```python
from build123d import *

# Parameters (mm, degrees)
SKETCH_W             = 18
SKETCH_H             = 25.7
PAD001_DEPTH         = 1
SKETCH002_R          = 1.1
PAD002_DEPTH         = 4.25
SKETCH004_W          = 20
SKETCH004_H          = 27.7
PAD004_DEPTH         = 8.5
SKETCH005_W          = 16
SKETCH005_H          = 0.5
POCKET_DEPTH         = 13.851
POCKET_DEPTH_BACK    = 13.851
SKETCH006_W          = 23.7
SKETCH006_H          = 0.5
POCKET001_DEPTH      = 10.001
POCKET001_DEPTH_BACK = 10.001
SKETCH007_W          = 18.8
SKETCH007_H          = 26.5
POCKET002_DEPTH      = 1


with BuildPart() as body004:
    # Sketch → Pad001 (new body)
    with BuildSketch(Plane.XY):
        Rectangle(SKETCH_W, SKETCH_H)
    extrude(amount=PAD001_DEPTH)

    # Sketch002 → Pad002 (join)
    with BuildSketch(Plane.XY):
        with Locations((5.556277, -9.06)):
            Circle(SKETCH002_R)
        Polygon((1.664554, 10.16), (1.400063, 8.66), (-2.320768, 8.66), (-2.950092, 9.41), (-2.056277, 10.16), align=None)
        Polygon((1.91841, 10.16), (1.65392, 8.66), (5.343461, 8.66), (6.237276, 9.41), (5.607952, 10.16), align=None)
        Polygon((-3.141603, 9.249303), (-2.512279, 8.499303), (-3.840514, 0.966506), (-4.734329, 0.216506), (-5.317726, 1.226979), (-4.035419, 8.499303), align=None)
        Polygon((6.397973, 9.218489), (5.504158, 8.468489), (4.217444, 1.171169), (4.80084, 0.160697), (5.694655, 0.910697), (7.027298, 8.468489), align=None)
        Polygon((-3.715514, 0.75), (-4.609329, 0), (-4.176316, -0.75), (-0.259174, -0.75), (0.005317, 0.75), align=None)
        Polygon((0.259174, 0.75), (-0.005317, -0.75), (3.715514, -0.75), (4.609329, 0), (4.176316, 0.75), align=None)
        Polygon((4.734329, -0.216506), (3.840514, -0.966506), (2.512279, -8.499303), (3.141603, -9.249303), (4.035419, -8.499303), (5.317726, -1.226979), align=None)
        Polygon((-4.217444, -1.171169), (-4.80084, -0.160697), (-5.694655, -0.910697), (-7.027298, -8.468489), (-6.397973, -9.218489), (-5.504158, -8.468489), align=None)
        Polygon((-5.343461, -8.66), (-6.237276, -9.41), (-5.607952, -10.16), (-1.91841, -10.16), (-1.65392, -8.66), align=None)
        Polygon((-1.400063, -8.66), (-1.664554, -10.16), (2.056277, -10.16), (2.950092, -9.41), (2.320768, -8.66), align=None)
        Polygon((-0.946713, -1.05), (0.576427, -1.05), (-0.712524, -8.36), (-2.235664, -8.36), align=None)
        Polygon((-0.576427, 1.05), (0.946713, 1.05), (2.235664, 8.36), (0.712524, 8.36), align=None)
        Polygon((-2.223397, 8.41), (-2.719177, 5.598295), (-0.889871, 1), (-0.394092, 3.811705), align=None)
        Polygon((1.791361, 4.112606), (1.242525, 1), (4.640381, 5.297394), (5.189217, 8.41), align=None)
        Polygon((0.889871, -1), (0.394092, -3.811705), (2.223397, -8.41), (2.719177, -5.598295), align=None)
        Polygon((-1.242525, -1), (-1.791361, -4.112606), (-5.189217, -8.41), (-4.640381, -5.297394), align=None)
    extrude(amount=PAD002_DEPTH)


with BuildPart() as body004_1:
    # Body001 placement: moved
    add(body004.part.moved(Location((0, 0, 4.25))))


with BuildPart() as obj1:
    # Sketch004 → Pad004 (new body)
    with BuildSketch(Plane.XY):
        Rectangle(SKETCH004_W, SKETCH004_H)
    extrude(amount=PAD004_DEPTH)

    # Sketch005 → Pocket (cut, two sides)
    with BuildSketch(Plane.XZ) as pocket_sk:
        with Locations((0, 0.25)):
            Rectangle(SKETCH005_W, SKETCH005_H)
    extrude(amount=-POCKET_DEPTH, mode=Mode.SUBTRACT)
    extrude(pocket_sk.sketch, amount=POCKET_DEPTH_BACK, mode=Mode.SUBTRACT)

    # Sketch006 → Pocket001 (cut, two sides)
    with BuildSketch(Plane.YZ) as pocket001_sk:
        with Locations((0, 0.25)):
            Rectangle(SKETCH006_W, SKETCH006_H)
    extrude(amount=-POCKET001_DEPTH, mode=Mode.SUBTRACT)
    extrude(pocket001_sk.sketch, amount=POCKET001_DEPTH_BACK, mode=Mode.SUBTRACT)

    # Sketch007 → Pocket002 (cut)
    with BuildSketch(Plane.XY):
        Rectangle(SKETCH007_W, SKETCH007_H)
    extrude(amount=POCKET002_DEPTH, mode=Mode.SUBTRACT)

    # Cut: cut Body004
    add(body004_1.part, mode=Mode.SUBTRACT)


solid = obj1.part
```
Source: CAD feature listing. Evaluate the final solid. Frame: model axes, mm. A direction names the side the tool comes from. Round coordinates to 2 decimals unless told otherwise and drop trailing zeros. Loops run counter-clockwise (first coordinate to the right, second up) from the corner with the lowest first, then second, coordinate; pieces in that order, holes last.
1. Contact query for flat-ended pins moving along their axis: pin 1 (9.5 mm diameter, centred on x = -0.5, y = -0.5, fed in from -Z); pin 2 (5 mm diameter, centred on x = 0, y = -1.5, fed in from +Z). Output: stop coordinate, or through.
2. Access query for faces 1 (the flat face through (0, 8.66, 7)), 2 (the flat face through (-0.1, 13.25, 0.7)), 3 (the flat face through (0, 0, 4.25)), 4 (the flat face through (9.7, 13.1, 0)). Directions: +Z, -Z, +X, -X, +Y, -Y. A direction counts if a zero-diameter tool reaches every point of the face in a straight line with its end or side. Return the directions, or none.
3. Section query A-A on y = 11. Output: boundary loops of the cut face in (x, z).
4. Section query B-B on z = 7.75. Give the number of separate pieces and of enclosed holes in the cut face, and give its area (3 significant figures).
5. Mould query, pull axis Y, two halves, no side actions, for faces 5 (the flat face through (-1.788, -9.42, 6.852)), 6 (the flat face through (-2, 3, 8.5)), 7 (the flat face through (0, -1.05, 7)). Classes: released by +Y, released by -Y, zero draft, split by the parting line, or undercut.
6. Ray query, L1, parallel to Z at x = -8, y = -6.75; L2, parallel to X at y = 7, z = 6.5; L3, parallel to X at y = -3.5, z = 7. Return the intervals inside material, ascending.
Answers below:
1. pin 1: stops at z = 1
1. pin 2: stops at z = 8.5
2. face 1: +Z
2. face 2: -Z
2. face 3: none
2. face 4: -Z, +X, -X, +Y, -Y
3. outline: (-10, 0.5) - (-9.4, 0.5) - (-9.4, 1) - (9.4, 1) - (9.4, 0.5) - (10, 0.5) - (10, 8.5) - (-10, 8.5) - close; hole (-9, 4.25) - (9, 4.25) - (9, 5.25) - (-9, 5.25) - close
4. separate pieces: 1
4. enclosed holes: 17
4. area: 410 mm2
5. face 5: undercut
5. face 6: zero draft
5. face 7: undercut
6. L1: z = 1 to 4.25, 5.25 to 8.5
6. L2: x = -10 to -4.3, -2.78 to -2.47, -1.66 to 0.47, 2 to 4.07, 4.94 to 5.25, 6.77 to 10
6. L3: x = -10 to -6.15, -4.63 to -3.22, -1.68 to -1.38, 0.14 to 0.45, 1.88 to 3.39, 4.92 to 10
